from build123d import *

# Parameters (mm, degrees)
SKETCH1_W               = 110.236
SKETCH1_H               = 72.136
RADIO_MOUNT_PLATE_DEPTH = 1.27
SKETCH2_R               = 1.95
SKETCH2_R_2             = 1.651
CUT_EXTRUDE1_DEPTH      = 132.746692907
SKETCH3_W               = 110.236
SKETCH3_H               = 2.54
BOSS_EXTRUDE2_DEPTH     = 23.37054
SKETCH4_R               = 2.286
CUT_EXTRUDE2_DEPTH      = 134.79746011
SKETCH5_W               = 76
SKETCH5_H               = 2.54
BOSS_EXTRUDE3_DEPTH     = 10
CHAMFER1_SIZE           = 1.27
CHAMFER2_SIZE           = 2.54


with BuildPart() as part:
    # Sketch1 → Radio Mount Plate (new body)
    with BuildSketch(Plane(origin=(0, 0, 0), x_dir=(1, 0, 0), z_dir=(0, 1, 0))):
        with Locations((55.118, 36.068)):
            Rectangle(SKETCH1_W, SKETCH1_H)
    extrude(amount=RADIO_MOUNT_PLATE_DEPTH)

    # Sketch2 → Cut-Extrude1 (cut, through all)
    with BuildSketch(Plane(origin=(0, 1.27, 0), x_dir=(1, 0, 0), z_dir=(0, 1, 0))):
        with Locations(Location((107.786, 59.368, 0), (0, 0, 270))):
            Circle(SKETCH2_R)
        with Locations(Location((38.036, 17.318, 0), (0, 0, 270))):
            Circle(SKETCH2_R)
        with Locations(Location((2.54, 53.848, 0), (0, 0, 270))):
            Circle(SKETCH2_R_2)
        with Locations(Location((30.48, 53.848, 0), (0, 0, 270))):
            Circle(SKETCH2_R_2)
        with Locations(Location((30.48, 18.288, 0), (0, 0, 270))):
            Circle(SKETCH2_R_2)
        with Locations(Location((2.54, 18.288, 0), (0, 0, 270))):
            Circle(SKETCH2_R_2)
    extrude(amount=-CUT_EXTRUDE1_DEPTH, mode=Mode.SUBTRACT)

    # Sketch3 → Boss-Extrude2 (add)
    with BuildSketch(Plane(origin=(0, 1.27, 0), x_dir=(1, 0, 0), z_dir=(0, 1, 0))):
        with Locations((55.118, 70.866)):
            Rectangle(SKETCH3_W, SKETCH3_H)
        with Locations((55.118, 1.27)):
            Rectangle(SKETCH3_W, SKETCH3_H)
    extrude(amount=BOSS_EXTRUDE2_DEPTH)

    # Sketch4 → Cut-Extrude2 (cut, through all)
    with BuildSketch(Plane(origin=(0, 1.27, 0), x_dir=(1, 0, 0), z_dir=(0, 1, 0))):
        with Locations(Location((6.35, 65.786, 0), (0, 0, 270))):
            Circle(SKETCH4_R)
        with Locations(Location((6.35, 6.35, 0), (0, 0, 90))):
            Circle(SKETCH4_R)
    extrude(amount=-CUT_EXTRUDE2_DEPTH, mode=Mode.SUBTRACT)

    # Sketch5 → Boss-Extrude3 (add)
    with BuildSketch(Plane(origin=(0, 1.27, 0), x_dir=(1, 0, 0), z_dir=(0, 1, 0))):
        with Locations((72.236, 64.358)):
            Rectangle(SKETCH5_W, SKETCH5_H)
        with Locations((72.236, 7.778)):
            Rectangle(SKETCH5_W, SKETCH5_H)
    extrude(amount=BOSS_EXTRUDE3_DEPTH)

    # Chamfer1
    chamfer1_edges = [part.edges().sort_by_distance(p)[0] for p in [
        (34.236, 11.27, -64.358),
        (72.236, 11.27, -63.088),
        (110.236, 11.27, -64.358),
        (72.236, 11.27, -65.628),
        (34.236, 11.27, -7.778),
        (72.236, 11.27, -6.508),
        (110.236, 11.27, -7.778),
        (72.236, 11.27, -9.048),
    ]]
    chamfer(chamfer1_edges, length=CHAMFER1_SIZE - 0.0001)  # a hair under: the kernel refuses the full size

    # Chamfer2
    chamfer2_edges = [part.edges().sort_by_distance(p)[0] for p in [
        (110.236, 12.32027, 0),
        (110.236, 12.32027, -72.136),
        (0, 12.32027, -72.136),
        (0, 12.32027, 0),
    ]]
    chamfer(chamfer2_edges, length=CHAMFER2_SIZE - 0.0001)  # a hair under: the kernel refuses the full size


solid = part.part
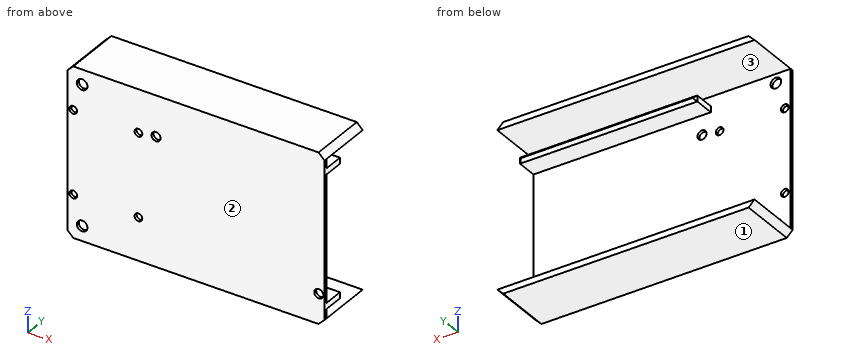
Geometry check sheet. Reference: the model listing, model coordinates, mm. Face numbers are marked on the shaded views. Give positions to 0.01 mm unless a question says otherwise; leave off trailing zeros. Order: outer loops, then holes, each group sorted by start corner. A loop starts at its lowest first (then second) coordinate and runs counter-clockwise, first axis right, second up.
1. Depth check by flat-ended pin: pin 1 (2.5 mm diameter, centred on x = 107.786, z = -59.368, fed in from +Y); pin 2 (1.5 mm diameter, centred on x = 50.5, z = -45.5, fed in from +Y); pin 3 (2 mm diameter, centred on y = 5.5, z = -8, fed in from -X). Enter the tip coordinate at first touch or a pass-through.
Completed:
pin 1: passes through
pin 2: stops at y = 1.27
pin 3: stops at x = 34.24
2. Scan lines: line 1 (Z direction, x = 85, y = 4.75); line 2 (Z direction, x = 78, y = 14.5); line 3 (Y direction, x = 9, z = -35). Record each from-to range of solid material in increasing order.
Completed:
line 1: z = -72.14 to -69.6, -65.63 to -63.09, -9.05 to -6.51, -2.54 to 0
line 2: z = -72.14 to -69.6, -2.54 to 0
line 3: y = 0 to 1.27
3. Draft check along Z on the marked faces 1, 2 and 3. Enter one of: pulls with the +Z half, pulls with the -Z half, needs draft (parallel to the pull), parting line crosses it, or undercut.
Completed:
face 1: pulls with the -Z half
face 2: needs draft
face 3: undercut
4. Sectioned sample at B-B (x = 6.35). Record the boundary of the cut face in (y, z).
Completed:
outline: (0, -72.14) - (24.64, -72.14) - (24.64, -69.6) - (1.27, -69.6) - (1.27, -68.07) - (0, -68.07) - close; (0, -63.5) - (1.27, -63.5) - (1.27, -8.64) - (0, -8.64) - close; (0, -4.06) - (1.27, -4.06) - (1.27, -2.54) - (24.64, -2.54) - (24.64, 0) - (0, 0) - close
5. Sectioned sample at D-D (x = 30.48). Record the boundary of the cut face in (y, z).
Completed:
outline: (0, -72.14) - (24.64, -72.14) - (24.64, -69.6) - (1.27, -69.6) - (1.27, -55.5) - (0, -55.5) - close; (0, -52.2) - (1.27, -52.2) - (1.27, -19.94) - (0, -19.94) - close; (0, -16.64) - (1.27, -16.64) - (1.27, -2.54) - (24.64, -2.54) - (24.64, 0) - (0, 0) - close
6. Sectioned sample at A-A (y = 6.5). State how many separate pieces and enclosed holes the cut face has, then the cut area to 3 significant figures.
Completed:
separate pieces: 4
enclosed holes: 0
area: 933 mm2
